Source: CAD feature listing. Evaluate the final solid. Frame: model axes, mm. Give positions to 0.01 mm unless a question says otherwise; leave off trailing zeros. Write each loop counter-clockwise with the first axis right and the second up, starting at its lowest first coordinate (ties: lowest second). Pieces come first, ordered by that corner, then holes. Notation, with made-up numbers: M 82.5,52.25 L 141.5,52.25 A24 ccw 141.5,88.25 Z; hole C 75.5,21.5 d9. An arc over 180 degrees is marked long. Answer as a JSON object with one key per item and string values. Group by question number.
```python
from build123d import *

# Parameters (mm, degrees)
SKETCH1_R           = 12.7
BOSS_EXTRUDE1_DEPTH = 165.1
SKETCH2_W           = 0.7874
SKETCH2_H           = 2.1844
CHAMFER1_SIZE       = 1.905


with BuildPart() as part:
    # Sketch1 → Boss-Extrude1 (new body)
    with BuildSketch(Plane.XY):
        Circle(SKETCH1_R)
    extrude(amount=BOSS_EXTRUDE1_DEPTH)

    # Sketch2 → Cut-Revolve1 (revolve, cut)
    with BuildSketch(Plane(origin=(0, 0, 0), x_dir=(1, 0, 0), z_dir=(0, 1, 0))):
        with Locations((-12.3063, -5.2578)):
            Rectangle(SKETCH2_W, SKETCH2_H)
        with Locations((-12.3063, -159.8422)):
            Rectangle(SKETCH2_W, SKETCH2_H)
    revolve(axis=Axis((0, 0, 0), (0, 0, 1)), mode=Mode.SUBTRACT)

    # Chamfer1
    chamfer1_edges = [part.edges().sort_by_distance(p)[0] for p in [
        (-12.7, 0, 0),
        (-12.7, 0, 165.1),
    ]]
    chamfer(chamfer1_edges, length=CHAMFER1_SIZE)


solid = part.part
```
(1) Ray query, L1, parallel to Z at x = -11.5, y = 5.25; L2, parallel to Z at x = -10, y = 7.5 (3 decimals); L3, parallel to X at y = -0.25, z = 146.5. Return the intervals inside material, ascending. Write a range as [from, to].
(2) Pull-direction query (Z, two-part tool) for faces 1 (the cylindrical face through (9.45, 7.25, 159.83)), 2 (the cylindrical face through (9.45, 7.25, 5.24)), 3 (the flat face through (0, 0, 165.1)), 4 (the cylindrical face through (-2.75, -12.4, 162.05)); classes: pulls with the +Z half, pulls with the -Z half, needs draft (parallel to the pull), parting line crosses it, or undercut.
(3) Section A-A, the plane z = 38.5. Return loops of the section in (x, y).
(4) Contact query for flat-ended pins moving along their axis: pin 1 Ø2 at (y, z) = (-8.5, 73) entering from +X; pin 2 Ø1 at (y, z) = (-9, 88) entering from +X; pin 3 Ø3 at (x, z) = (-7, 138) entering from +Y. Output: stop coordinate, or through.
Reported:
{
 "1": {"L1": "z = [1.85, 4.17], [6.35, 158.75], [160.93, 163.25]", "L2": "z = [1.705, 4.166], [6.35, 158.75], [160.934, 163.395]", "L3": "x = [-12.7, 12.7]"},
 "2": {"face 1": "undercut", "face 2": "undercut", "face 3": "pulls with the +Z half", "face 4": "needs draft"},
 "3": {"outline": "C 0,0 d25.4"},
 "4": {"pin 1": "stops at x = 10.25", "pin 2": "stops at x = 9.44", "pin 3": "stops at y = 11.45"}
}
